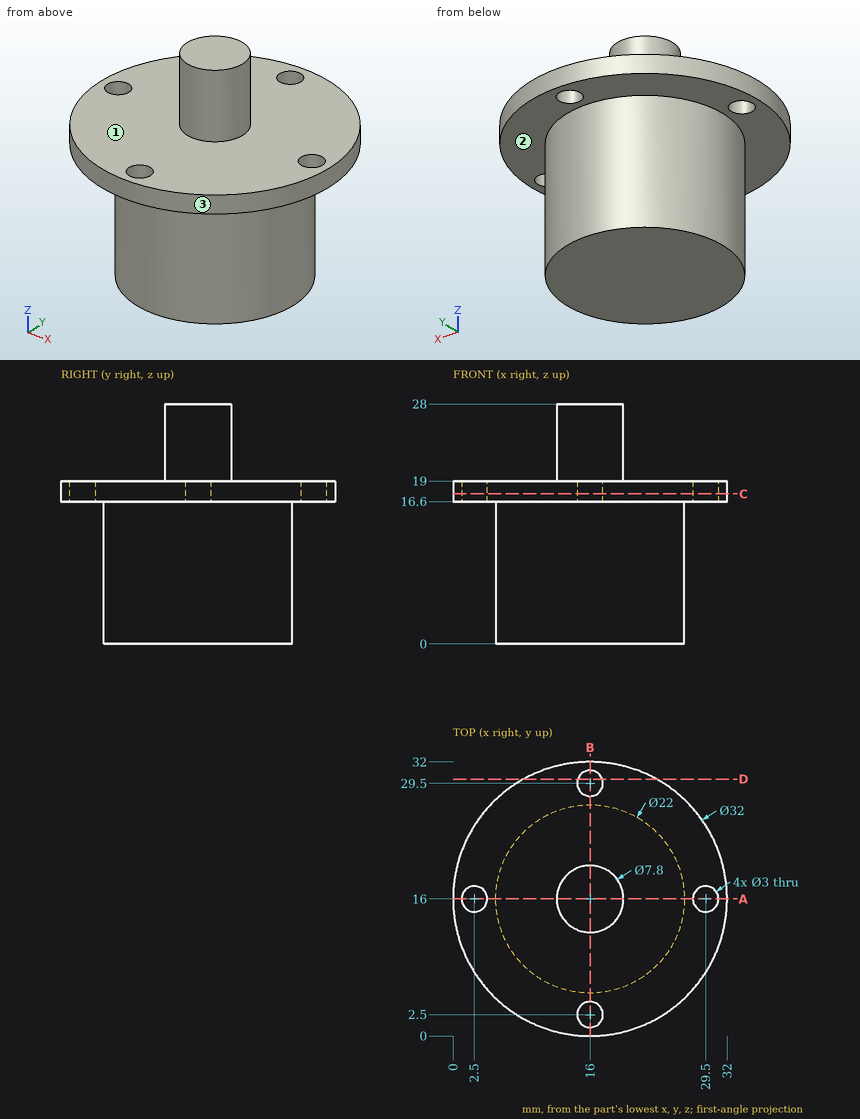
Print and shaded views of the part. All mm, measured from the part's lowest x, y and z. A direction names the side the tool comes from. Coordinates: 2 decimals unless noted, no trailing zeros. Loops run counter-clockwise (first coordinate to the right, second up) from the corner with the lowest first, then second, coordinate; pieces in that order, holes last. Notation, with made-up numbers: (10, 58.25) - (39, 58.25) arc R14 ccw to (39, 79.25) - close; hole circle Ø7 at (-29.5, 82.25). An arc over 180 degrees is marked (long way). Write item = value, one per line. Start each with the question number.
Item 1: Cut at A-A, the plane y = 16. Give the cut face in (x, z), and give its area (3 significant figures).
Item 2: Cut at D-D, the plane y = 30. Give the cut face in (x, z).
Item 3: Wall check: L1, parallel to Y at x = 16, z = 17.1; L2, parallel to Z at x = 22, y = 15; L3, parallel to Z at x = 23, y = 4. Give the ranges that are in metal, low to high. Write a range as from..to.
Item 4: 3-axis set-ups, long thin cutter, end or side, ignore diameter. For the marked faces 1, 2 and 3: which of +Z, -Z, +X, -X, +Y, -Y reach the whole face in a straight line?
Item 5: Cut at C-C, the plane z = 17.5. Give the cut face in (x, y).
Item 6: Flat gauge pins, fed straight in: pin 1 Ø5 at (x, z) = (4, 18.5) entering from -Y; pin 2 Ø3 at (x, y) = (17.5, 21.5) entering from +Z; pin 3 Ø12 at (x, z) = (8, 8) entering from -Y; pin 4 Ø1 at (x, z) = (10.5, 20.5) entering from -Y. Where does each tip first touch, or does it go through?
The answers:
q1.outline = (0, 16.6) - (1, 16.6) - (1, 19) - (0, 19) - close; (4, 16.6) - (5, 16.6) - (5, 0) - (27, 0) - (27, 16.6) - (28, 16.6) - (28, 19) - (19.9, 19) - (19.9, 28) - (12.1, 28) - (12.1, 19) - (4, 19) - close; (31, 16.6) - (32, 16.6) - (32, 19) - (31, 19) - close
q1.area = 498 mm2
q2.outline = (8.25, 16.6) - (14.59, 16.6) - (14.59, 19) - (8.25, 19) - close; (17.41, 16.6) - (23.75, 16.6) - (23.75, 19) - (17.41, 19) - close
q3.L1 = 0..1, 4..28, 31..32
q3.L2 = 0..19
q3.L3 = 16.6..19
q4.face_1 = +Z
q4.face_2 = -Z
q4.face_3 = +Z, -Z
q5.outline = circle Ø32 at (16, 16); hole circle Ø3 at (2.5, 16); hole circle Ø3 at (16, 2.5); hole circle Ø3 at (16, 29.5); hole circle Ø3 at (29.5, 16)
q6.pin_1 = 3.13
q6.pin_2 = 19
q6.pin_3 = 5.18
q6.pin_4 = through
